Read the model definition and answer for the solid it produces. Units are mm, in the model's axes. A direction names the side the tool comes from. Coordinates: 2 decimals unless noted, no trailing zeros. Loops run counter-clockwise (first coordinate to the right, second up) from the corner with the lowest first, then second, coordinate; pieces in that order, holes last.
from build123d import *

# Parameters (mm, degrees)
F0_R     = 76.431145
F0_R_2   = 65
F1_DEPTH = 69
F0_W     = 170
F0_H     = 170
F2_DEPTH = 7
F4_DEPTH = 25


with BuildPart() as f1:
    # F0 (on Top) → F1 (new body)
    with BuildSketch(Plane.XY):
        Circle(F0_R)
        Circle(F0_R_2, mode=Mode.SUBTRACT)
    extrude(amount=F1_DEPTH)

    # F0 (on Top) → F2 (join)
    with BuildSketch(Plane.XY):
        Rectangle(F0_W, F0_H)
        Circle(F0_R, mode=Mode.SUBTRACT)
        Circle(F0_R)
        Circle(F0_R_2, mode=Mode.SUBTRACT)
    extrude(amount=-F2_DEPTH)

    # F3 (on face) → F4 (join)
    with BuildSketch(Plane.XY):
        with BuildLine():
            ThreePointArc((-46.036632, -61.011052), (-54.149607, -53.940152), (-61.189011, -45.799835))
            Line((-61.189011, -45.799835), (-83.201844, -62.276389))
            Line((-83.201844, -62.276389), (-63.29952, -83.889073))
            Line((-63.29952, -83.889073), (-46.036632, -61.011052))
        make_face()
    extrude(amount=F4_DEPTH)


solid = f1.part
Item 1: Which of the six approach directions +Z, -Z, +X, -X, +Y, -Y give full straight-line access (tool end or side, diameter ignored) to faces 4 (the face through (-1, 77, 0)), 5 (the face through (-73.39, -72.93, 12.32)), 6 (the face through (-1, 85, -3))?
Numbers:
face 4: +Z
face 5: +Z, -X, -Y
face 6: +Z, -Z, +X, -X, +Y
Item 2: A cutting plane is placed at C-C on z = 12.5. Determine the outline of the cut face in (x, y).
Numbers:
outline: (-83.2, -62.28) - (-63.3, -83.89) - (-46.04, -61.01) arc R76.43 ccw (long way) to (-61.19, -45.8) - close; hole circle Ø130 at (0, 0)
Item 3: A cutting plane is placed at A-A on x = 0. Determine the outline of the cut face in (y, z).
Numbers:
outline: (-85, -7) - (-65, -7) - (-65, 69) - (-76.43, 69) - (-76.43, 0) - (-85, 0) - close; (65, -7) - (85, -7) - (85, 0) - (76.43, 0) - (76.43, 69) - (65, 69) - close
Item 4: Determine the mould class of faces 1 (the face through (-72.04, -53.92, 12.32)), 2 (the face through (-54.79, -72.61, 12.32)), 3 (the face through (-58, -37, -7)) for opening direction Y: released by +Y, released by -Y, zero draft, split by the parting line, or undercut.
Numbers:
face 1: undercut
face 2: released by -Y
face 3: zero draft
Item 5: Find the intervals of material crossed by line 1 along Y through (x, z) = (0, 49); line 2 along Y through (x, z) = (0, -5); line 3 along Z through (x, y) = (-20, 74.5), in increasing order.
Numbers:
line 1: y = -76.43 to -65, 65 to 76.43
line 2: y = -85 to -65, 65 to 85
line 3: z = -7 to 0
Item 6: Given pin 1 (5 mm diameter, centred on y = -44.5, z = 25.5, fed in from +X); pin 2 (6 mm diameter, centred on x = -39, z = 22.5, fed in from -Y); pin 3 (4 mm diameter, centred on y = 62, z = 47, fed in from -X), each flat-ended and moving along its own axis, determine where each tip first touches the part or whether it passes through.
Numbers:
pin 1: stops at x = 63.86
pin 2: stops at y = -67.42
pin 3: stops at x = -47.35
Item 7: A cutting plane is placed at D-D on y = 68. Determine the outline of the cut face in (x, z), then the cut area to 3 significant figures.
Numbers:
outline: (-85, -7) - (85, -7) - (85, 0) - (34.9, 0) - (34.9, 69) - (-34.9, 69) - (-34.9, 0) - (-85, 0) - close
area: 6,010 mm2
